```python
from build123d import *

# Parameters (mm, degrees)
F0_W      = 69.85
F0_H      = 44.45
F1_DEPTH  = 25.4
F3_DEPTH  = 25.4
F4_DEPTH  = 25.4
F6_DEPTH  = 31.75
F7_R      = 6.0952761175
F8_DEPTH  = 25.4
F9_R      = 5.6297266716
F10_DEPTH = 25.4
F12_DEPTH = 25.4
F13_R     = 5.87576174
F14_DEPTH = 25.4


with BuildPart() as f1:
    # F0 (on Front) → F1 (new body)
    with BuildSketch(Plane.XZ):
        with Locations((13.0522018299, -8.6590135922)):
            Rectangle(F0_W, F0_H)
    extrude(amount=F1_DEPTH)

    # F2 (on face) → F3 (cut)
    with BuildSketch(Plane.XY.offset(13.5659864078)):
        with BuildLine():
            Line((-21.8727981701, -25.4), (-12.6271519341, -25.4))
            ThreePointArc((-12.6271519341, -25.4), (-21.7253869392, -12.3045156894), (-11.5829768121, 0))
            Line((-11.5829768121, 0), (-21.8727981701, 0))
            Line((-21.8727981701, 0), (-21.8727981701, -25.4))
        make_face()
        with BuildLine():
            ThreePointArc((36.6770463917, 0), (47.8953651974, -12.4202974309), (37.3292975128, -25.4))
            Line((37.3292975128, -25.4), (47.9772018299, -25.4))
            Line((47.9772018299, -25.4), (47.9772018299, 0))
            Line((47.9772018299, 0), (36.6770463917, 0))
        make_face()
    extrude(amount=-F3_DEPTH, mode=Mode.SUBTRACT)

    # F4 (cut): faces of the model
    f4_faces = [f1.faces().sort_by_distance(p)[0] for p in [
        (-21.7527689283, -12.3033900362, -11.8340135922),
        (47.923156279, -12.4195837788, -11.8340135922),
    ]]
    extrude(f4_faces, amount=-F4_DEPTH, mode=Mode.SUBTRACT)

    # F5 (on face) → F6 (cut)
    with BuildSketch(Plane.XY.offset(13.5659864078)):
        with BuildLine():
            ThreePointArc((-12.6271519341, -0.2937349935), (-21.7365300731, -12.8468674968), (-12.6271519341, -25.4))
            Line((-12.6271519341, -25.4), (-12.6271519341, -0.2937349935))
        make_face()
        with BuildLine():
            Line((-12.6271519341, -0.2937349935), (-12.6271519341, -25.4))
            Line((-12.6271519341, -25.4), (0, -25.4))
            Line((0, -25.4), (0, 0))
            Line((0, 0), (-11.5829768121, 0))
            ThreePointArc((-11.5829768121, 0), (-12.1080819056, -0.136140711), (-12.6271519341, -0.2937349935))
        make_face()
        with BuildLine():
            Line((24.6292975128, 0), (24.6292975128, -25.4))
            Line((24.6292975128, -25.4), (37.3292975128, -25.4))
            Line((37.3292975128, -25.4), (37.3292975128, -0.1005509322))
            ThreePointArc((37.3292975128, -0.1005509322), (37.0038173622, -0.046088838), (36.6770463917, 0))
            Line((36.6770463917, 0), (24.6292975128, 0))
        make_face()
        with BuildLine():
            Line((37.3292975128, -0.1005509322), (37.3292975128, -25.4))
            ThreePointArc((37.3292975128, -25.4), (47.8996012815, -12.7502754661), (37.3292975128, -0.1005509322))
        make_face()
    extrude(amount=-F6_DEPTH, mode=Mode.SUBTRACT)

    # F7 (on face) → F8 (cut)
    with BuildSketch(Plane.XY.offset(-18.1840135922)):
        with Locations((-8.5324506041, -12.8468674968)):
            Circle(F7_R)
    extrude(amount=-F8_DEPTH, mode=Mode.SUBTRACT)

    # F9 (on face) → F10 (cut)
    with BuildSketch(Plane.XY.offset(-18.1840135922)):
        with Locations((35.0453419106, -12.7502754661)):
            Circle(F9_R)
    extrude(amount=-F10_DEPTH, mode=Mode.SUBTRACT)

    # F11 (on face) → F12 (cut)
    with BuildSketch(Plane(origin=(0, 0, 0), x_dir=(0, -1, 0), z_dir=(-1, 0, 0))):
        with BuildLine():
            Line((0, 13.5659864078), (0, 0))
            ThreePointArc((0, 0), (12.7, 12.7), (25.4, 0))
            Line((25.4, 0), (25.4, 13.5659864078))
            Line((25.4, 13.5659864078), (0, 13.5659864078))
        make_face()
    extrude(amount=-F12_DEPTH, mode=Mode.SUBTRACT)

    # F13 (on face) → F14 (cut)
    with BuildSketch(Plane(origin=(0, 0, 0), x_dir=(0, -1, 0), z_dir=(-1, 0, 0))):
        with Locations((12.7, 0)):
            Circle(F13_R)
    extrude(amount=-F14_DEPTH, mode=Mode.SUBTRACT)


solid = f1.part
```
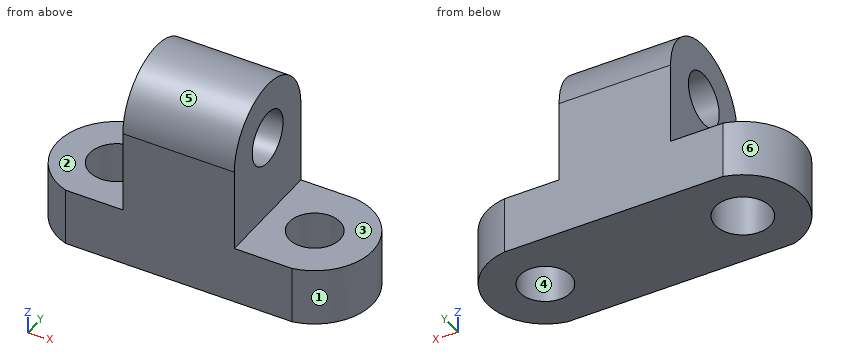
Input: part model. Units: mm. Frame: model coordinates. Face numbers are marked on the shaded views. A direction names the side the tool comes from. Give positions to 0.01 mm unless a question says otherwise; leave off trailing zeros. Write each loop counter-clockwise with the first axis right and the second up, starting at its lowest first coordinate (ties: lowest second). Pieces come first, ordered by that corner, then holes. Notation, with made-up numbers: (6, 41.25) - (35, 41.25) arc R34 ccw to (35, 78.25) - close; hole circle Ø11 at (76, 29.5). An arc over 180 degrees is marked (long way). Write item = value, one per line. Start each with the question number.
1. First-contact query: pin 1 Ø3 at (y, z) = (-19, -11.5) entering from +X; pin 2 Ø9.5 at (y, z) = (-12.7, 0) entering from -X; pin 3 Ø11.5 at (x, y) = (33, -6.5) entering from +Z; pin 4 Ø1 at (y, z) = (-21, -16) entering from -X. Flat tips, straight axial feed; report the tip coordinate or a pass-through.
2. Section query B-B, the plane x = 14. Output: boundary loops of the cut face in (y, z).
3. Access query for the marked faces 1, 2 and 3. Directions: +Z, -Z, +X, -X, +Y, -Y. A direction counts if a zero-diameter tool reaches every point of the face in a straight line with its end or side. Return the directions, or none.
4. Section query C-C, the plane y = -21. Output: boundary loops of the cut face in (x, z), then the cut area to 3 significant figures.
5. Section query D-D, the plane z = -19. Output: boundary loops of the cut face in (x, y), then the cut area to 3 significant figures.
6. Ray query, L1, parallel to Z at x = 6, y = -12.7; L2, parallel to X at y = -16.5, z = -24.5; L3, parallel to X at y = -17.75, z = -26. Return the intervals inside material, ascending.
7. Mould query, pull axis X, two halves, no side actions, for the marked faces 4, 5 and 6. Classes: released by +X, released by -X, zero draft, split by the parting line, or undercut.
8. Section query A-A, the plane z = 5. Output: boundary loops of the cut face in (x, y), then the cut area to 3 significant figures.
Check sheet entries:
q1.pin_1 = 24.63
q1.pin_2 = through
q1.pin_3 = -18.18
q1.pin_4 = 0
q2.outline = (-25.4, -30.88) - (0, -30.88) - (0, 0) arc R12.7 ccw to (-25.4, 0) - close; hole circle Ø11.75 at (-12.7, 0)
q3.face_1 = +Z, -Z, +X
q3.face_2 = +Z, -X, +Y, -Y
q3.face_3 = +Z, +X, +Y, -Y
q4.outline = (-18.92, -30.88) - (44.9, -30.88) - (44.9, -18.18) - (24.63, -18.18) - (24.63, 9.61) - (0, 9.61) - (0, -18.18) - (-18.92, -18.18) - close
q4.area = 1,500 mm2
q5.outline = (-12.63, -25.4) - (37.33, -25.4) arc R12.85 ccw to (36.68, 0) - (-11.58, 0) arc R13.2 ccw to start; hole circle Ø12.19 at (-8.53, -12.85); hole circle Ø11.26 at (35.05, -12.75)
q5.area = 1,420 mm2
q6.L1 = -30.88 to -5.88, 5.88 to 12.7
q6.L2 = -21.22 to -13.41, -3.65 to 30.85, 39.24 to 47.34
q6.L3 = -20.79 to -12.15, -4.91 to 32.46, 37.63 to 46.89
q7.face_4 = undercut
q7.face_5 = zero draft
q7.face_6 = released by -X
q8.outline = (0, -24.37) - (24.63, -24.37) - (24.63, -15.79) - (0, -15.79) - close; (0, -9.61) - (24.63, -9.61) - (24.63, -1.03) - (0, -1.03) - close
q8.area = 423 mm2
